from build123d import *

# Parameters (mm, degrees)
SKETCH1_W           = 20
SKETCH1_H           = 20
SKETCH1_R           = 1.6
BOSS_EXTRUDE1_DEPTH = 4
SKETCH2_W           = 20
SKETCH2_H           = 4
BOSS_EXTRUDE2_DEPTH = 19
FILLET1_R           = 3
FILLET2_R           = 5


with BuildPart() as part:
    # Sketch1 → Boss-Extrude1 (new body)
    with BuildSketch(Plane(origin=(0, 0, 0), x_dir=(1, 0, 0), z_dir=(0, 1, 0))):
        with Locations((10, -10)):
            Rectangle(SKETCH1_W, SKETCH1_H)
        with Locations(Location((10, -10, 0), (0, 0, 270))):
            Circle(SKETCH1_R, mode=Mode.SUBTRACT)
    extrude(amount=BOSS_EXTRUDE1_DEPTH)

    # Sketch2 → Boss-Extrude2 (add)
    with BuildSketch(Plane(origin=(0, 0, 0), x_dir=(-1, 0, 0), z_dir=(0, -1, 0))):
        with Locations((-10, -22)):
            Rectangle(SKETCH2_W, SKETCH2_H)
    extrude(amount=-BOSS_EXTRUDE2_DEPTH)

    # Fillet1
    fillet1_edges = [part.edges().sort_by_distance(p)[0] for p in [
        (10, 4, 20),
    ]]
    fillet(fillet1_edges, radius=FILLET1_R)

    # Fillet2
    fillet2_edges = [part.edges().sort_by_distance(p)[0] for p in [
        (0, 2, 0),
        (20, 2, 0),
    ]]
    fillet(fillet2_edges, radius=FILLET2_R)


solid = part.part
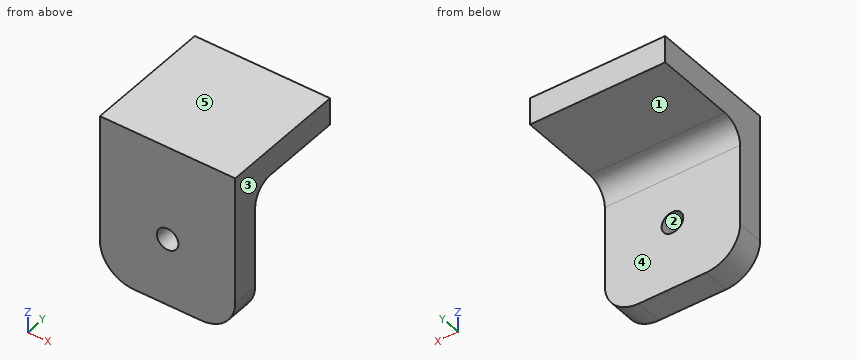
The model under review builds one solid part; all positions refer to its coordinate system, in mm. Face numbers are marked on the shaded views. A direction names the side the tool comes from. Round coordinates to 2 decimals unless told otherwise and drop trailing zeros. Loops run counter-clockwise (first coordinate to the right, second up) from the corner with the lowest first, then second, coordinate; pieces in that order, holes last. Notation, with made-up numbers: (47, 31) -> (58, 31) arc R22 cw to (58, 70) -> close; hole circle Ø10 at (87.25, 74.25). An arc over 180 degrees is marked (long way). Answer as CSV lines item,"result".
1) Draft analysis for pull direction Z (two halves, no side actions). For the marked faces 1, 2 and 3, state which applies: pulls with the +Z half, pulls with the -Z half, needs draft (parallel to the pull), parting line crosses it, or undercut.
Geometry results:
face 1,"pulls with the -Z half"
face 2,"undercut"
face 3,"needs draft"
2) Add section A-A on x = 10. Write out the cut boundary in (y, z).
Geometry results:
outline,"(0, 0) -> (4, 0) -> (4, 8.4) -> (0, 8.4) -> close; (0, 11.6) -> (4, 11.6) -> (4, 17) arc R3 cw to (7, 20) -> (19, 20) -> (19, 24) -> (0, 24) -> close"
3) Add section D-D on z = 1.5. Write out the cut boundary in (x, y).
Geometry results:
outline,"(1.43, 0) -> (18.57, 0) -> (18.57, 4) -> (1.43, 4) -> close"
4) To check wall thickness, follow line 1 along X through (y, z) = (1.7, 10); line 2 along Z through (x, y) = (6.5, 12); line 3 along Y through (x, z) = (10, 4.5). State the ranges of each line that lie inside material, in increasing order. Write a range as from..to.
Geometry results:
line 1,"x = 0..8.4, 11.6..20"
line 2,"z = 20..24"
line 3,"y = 0..4"
5) For P1, Ø3, axis at y = 6.5, z = 2.5, coming from the +X side; P2, Ø6, axis at x = 13.5, y = 13, coming from the -Z side; P3, Ø6, axis at x = 4, z = 16, coming from the +Y side, all flat-tipped, find the tip position at first contact; note any pin that passes through.
Geometry results:
P1,"passes through"
P2,"stops at z = 20"
P3,"stops at y = 4.76"
6) Add section B-B on z = 10. Write out the cut boundary in (x, y), plus the area to 3 significant figures.
Geometry results:
outline,"(0, 0) -> (8.4, 0) -> (8.4, 4) -> (0, 4) -> close; (11.6, 0) -> (20, 0) -> (20, 4) -> (11.6, 4) -> close"
area,"67.2 mm²"
7) Tool access review of the marked faces 4 and 5: name each direction out of +Z, -Z, +X, -X, +Y, -Y from which nothing blocks a thin tool from reaching the whole face with its end or side.
Geometry results:
face 4,"-Z, +X, -X, +Y"
face 5,"+Z, +X, -X, +Y, -Y"
8) Add section C-C on x = 7. Write out the cut boundary in (y, z), plus the area to 3 significant figures.
Geometry results:
outline,"(0, 0) -> (4, 0) -> (4, 17) arc R3 cw to (7, 20) -> (19, 20) -> (19, 24) -> (0, 24) -> close"
area,"158 mm²"
